```python
from build123d import *

# Parameters (mm, degrees)
SKETCH2_R          = 25
SKETCH1_R          = 22
SHELL1_T           = -2
SKETCH3_R          = 3
SKETCH3_R_2        = 2
SKETCH3_R_3        = 4
SKETCH3_R_4        = 1.3
CUT_EXTRUDE1_DEPTH = 37.362755832
CUT_EXTRUDE2_DEPTH = 31
CIRPATTERN1_COUNT  = 4
SKETCH5_R          = 5
CUT_EXTRUDE3_DEPTH = 0.5


with BuildPart() as part:
    # Sketch2 → Loft1 section 0
    with BuildSketch(Plane(origin=(0, 8.5, 0), x_dir=(1, 0, 0), z_dir=(0, 1, 0))):
        Circle(SKETCH2_R)
    # Sketch1 → Loft1 section 1
    with BuildSketch(Plane(origin=(0, 0, 0), x_dir=(1, 0, 0), z_dir=(0, 1, 0))):
        Circle(SKETCH1_R)
    loft()

    # Shell1
    shell1_openings = [part.faces().sort_by_distance(p)[0] for p in [
        (0, 8.5, 0),
    ]]
    offset(amount=SHELL1_T, openings=shell1_openings, kind=Kind.INTERSECTION)

    # Sketch3 → Cut-Extrude1 (cut, through all)
    with BuildSketch(Plane.XZ):
        with Locations(Location((0, 0, 0), (0, 0, 270))):
            Circle(SKETCH3_R)
        with Locations(Location((0, -12.25, 0), (0, 0, 270))):
            Circle(SKETCH3_R_2)
        with Locations(Location((-12.25, 0, 0), (0, 0, 270))):
            Circle(SKETCH3_R_2)
        with Locations(Location((0, 12.25, 0), (0, 0, 270))):
            Circle(SKETCH3_R_2)
        with Locations(Location((12.25, 0, 0), (0, 0, 270))):
            Circle(SKETCH3_R_2)
        with Locations(Location((-10.606601718, -10.606601718, 0), (0, 0, 270))):
            Circle(SKETCH3_R_3)
        with Locations(Location((-10.606601718, 10.606601718, 0), (0, 0, 270))):
            Circle(SKETCH3_R_3)
        with Locations(Location((10.606601718, 10.606601718, 0), (0, 0, 270))):
            Circle(SKETCH3_R_3)
        with Locations(Location((10.606601718, -10.606601718, 0), (0, 0, 270))):
            Circle(SKETCH3_R_3)
        with Locations(Location((-7.5, 0, 0), (0, 0, 270))):
            Circle(SKETCH3_R_4)
        with Locations(Location((3.75, 6.495190528, 0), (0, 0, 270))):
            Circle(SKETCH3_R_4)
        with Locations(Location((3.75, -6.495190528, 0), (0, 0, 270))):
            Circle(SKETCH3_R_4)
    extrude(amount=-CUT_EXTRUDE1_DEPTH, mode=Mode.SUBTRACT)

    # Sketch4 → Cut-Extrude2 (cut)
    with BuildSketch(Plane.XY):
        with BuildLine():
            Line((5, 2.2), (-5, 2.2))
            ThreePointArc((-5, 2.2), (-6.8, 4), (-5, 5.8))
            Line((-5, 5.8), (5, 5.8))
            ThreePointArc((5, 5.8), (6.8, 4), (5, 2.2))
        make_face()
    cut_extrude2 = extrude(amount=CUT_EXTRUDE2_DEPTH, mode=Mode.SUBTRACT)

    # CirPattern1: Cut-Extrude2 ×4 about axis
    cirpattern1_axis = Axis((0, 0, 0), (0, 1, 0))
    for i in range(1, CIRPATTERN1_COUNT):
        add(cut_extrude2.rotate(cirpattern1_axis, i * 360 / CIRPATTERN1_COUNT), mode=Mode.SUBTRACT)

    # Sketch5 → Cut-Extrude3 (cut)
    with BuildSketch(Plane.XZ):
        with Locations(Location((0, 0, 0), (0, 0, 270))):
            Circle(SKETCH5_R)
    extrude(amount=-CUT_EXTRUDE3_DEPTH, mode=Mode.SUBTRACT)


solid = part.part
```
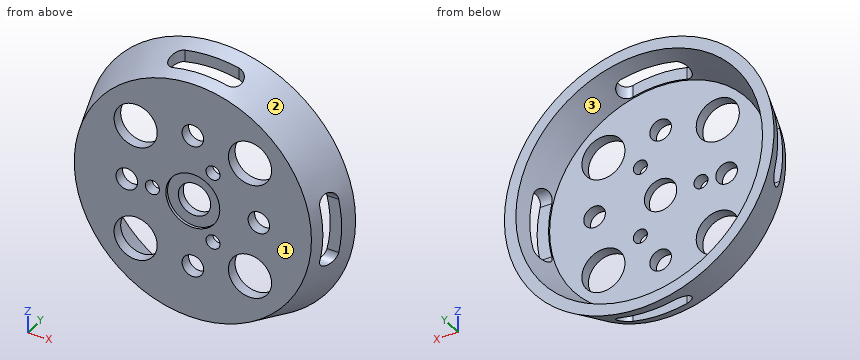
Part model, mm, in its own coordinate system. Face numbers are marked on the shaded views. Round coordinates to 2 decimals unless told otherwise and drop trailing zeros. Loops run counter-clockwise (first coordinate to the right, second up) from the corner with the lowest first, then second, coordinate; pieces in that order, holes last.
1. Slice it at A-A (y = 4). Give the cut face in (x, z), and give its area (3 significant figures).
Solutions:
outline: (-22.4, -6.8) arc R23.41 ccw to (-6.8, -22.4) - (-6.8, -20.18) arc R21.29 cw to (-20.18, -6.8) - close; (-22.4, 6.8) - (-20.18, 6.8) arc R21.29 cw to (-6.8, 20.18) - (-6.8, 22.4) arc R23.41 ccw to start; (6.8, -22.4) arc R23.41 ccw to (22.4, -6.8) - (20.18, -6.8) arc R21.29 cw to (6.8, -20.18) - close; (6.8, 20.18) arc R21.29 cw to (20.18, 6.8) - (22.4, 6.8) arc R23.41 ccw to (6.8, 22.4) - close
area: 181 mm2
2. Flat gauge pins, fed straight in: pin 1 (2 mm diameter, centred on x = -9.5, y = 5.5, fed in from +Z); pin 2 (7 mm diameter, centred on x = -10.61, z = 10.61, fed in from +Y); pin 3 (1.5 mm diameter, centred on x = -17, z = -14, fed in from -Y); pin 4 (1 mm diameter, centred on y = 2.5, z = 15, fed in from -X). Where does each tip first touch, or does it go through?
Solutions:
pin 1: stops at z = 22.54
pin 2: passes through
pin 3: stops at y = 0
pin 4: stops at x = -17.76
3. Drill centre lines: line 1 along X through (y, z) = (0.9, 12.25); line 2 along Z through (x, y) = (-9, 1.25); line 3 along Y through (x, z) = (-5.5, 9). Where is each one in solid material? Low to high.
Solutions:
line 1: x = -18.66 to -14.25, -6.96 to -2, 2 to 6.96, 14.25 to 18.66
line 2: z = -20.56 to -14.27, -6.94 to 6.94, 14.27 to 20.56
line 3: y = 0 to 2
4. Two-plate mould, pull along X, no slides. Class the marked faces 1, 2 and 3: pulls with the +X half, pulls with the -X half, needs draft (parallel to the pull), parting line crosses it, or undercut.
Solutions:
face 1: needs draft
face 2: parting line crosses it
face 3: undercut
5. Slice it at B-B (x = 0). Count the separate pieces of the cut face and the enclosed holes in it, and give its area (3 significant figures).
Solutions:
separate pieces: 6
enclosed holes: 0
area: 71.7 mm2
